Read the model definition and answer for the solid it produces. Units are mm, in the model's axes. Coordinates: 2 decimals unless noted, no trailing zeros. Loops run counter-clockwise (first coordinate to the right, second up) from the corner with the lowest first, then second, coordinate; pieces in that order, holes last.
from build123d import *

# Parameters (mm, degrees)
BOSS_EXTRUDE1_DEPTH          = 3
CUT_EXTRUDE_THIN1_DEPTH      = 73.819983521
CUT_EXTRUDE_THIN1_DEPTH_BACK = 3
FILLET1_R                    = 3.05
BOSS_EXTRUDE2_DEPTH          = 3
CUT_EXTRUDE1_DEPTH           = 77.32004979
CUT_EXTRUDE1_DEPTH_BACK      = 77.32004979
SKETCH4_R                    = 1.2
CUT_EXTRUDE_THIN2_DEPTH      = 77.32004979
CUT_EXTRUDE_THIN2_DEPTH_BACK = 3
FILLET2_R                    = 1.2
SKETCH6_W                    = 20
SKETCH6_H                    = 10
SKETCH6_R                    = 2.525
BOSS_EXTRUDE3_DEPTH          = 3
FILLET3_R                    = 3


with BuildPart() as part:
    # Sketch1 → Boss-Extrude1 (new body)
    with BuildSketch(Plane(origin=(0, 0, 0), x_dir=(1, 0, 0), z_dir=(0, 1, 0))):
        with BuildLine():
            Line((-27.5, 47.631397208), (-20.5, 35.507041555))
            ThreePointArc((-20.5, 35.507041555), (-40.649239316, 5.351573881), (-28.991378029, -28.991378029))
            Line((-28.991378029, -28.991378029), (-38.890872965, -38.890872965))
            ThreePointArc((-38.890872965, -38.890872965), (-54.529467376, 7.178940572), (-27.5, 47.631397208))
        make_face()
    extrude(amount=BOSS_EXTRUDE1_DEPTH)

    # Sketch2 → Cut-Extrude-Thin1 (cut, two sides: drawn at the far end of the back side and taken through both)
    with BuildSketch(Plane(origin=(0, 3, 0), x_dir=(1, 0, 0), z_dir=(0, 1, 0)).offset(-CUT_EXTRUDE_THIN1_DEPTH_BACK)):
        with BuildLine():
            ThreePointArc((-32.997630308, -29.03030992), (-43.925085447, -1.479651456), (-34.876429564, 26.743918204))
            Line((-34.876429564, 26.743918204), (-39.717071665, 30.455815838))
            ThreePointArc((-39.717071665, 30.455815838), (-50.021627455, -1.685018325), (-37.577506187, -33.0595452))
            Line((-37.577506187, -33.0595452), (-32.997630308, -29.03030992))
        make_face()
    extrude(amount=CUT_EXTRUDE_THIN1_DEPTH + CUT_EXTRUDE_THIN1_DEPTH_BACK, mode=Mode.SUBTRACT)

    # Fillet1
    fillet1_edges = [part.edges().sort_by_distance(p)[0] for p in [
        (-39.717071665, 1.5, -30.455815838),
        (-34.876429564, 1.5, -26.743918204),
        (-32.997630308, 1.5, 29.03030992),
        (-37.577506187, 1.5, 33.0595452),
    ]]
    fillet(fillet1_edges, radius=FILLET1_R - 0.0001)  # a hair under: the kernel refuses the full size

    # Sketch3 → Boss-Extrude2 (add)
    with BuildSketch(Plane(origin=(0, 0, 0), x_dir=(1, 0, 0), z_dir=(0, 1, 0))):
        with BuildLine():
            Line((-27.5, 47.631397208), (-30.5, 52.827549631))
            ThreePointArc((-30.5, 52.827549631), (-36.284189992, 49.035268498), (-41.601899964, 44.612575799))
            Line((-41.601899964, 44.612575799), (-37.509909803, 40.224453589))
            ThreePointArc((-37.509909803, 40.224453589), (-32.715253271, 44.212127334), (-27.5, 47.631397208))
        make_face()
    extrude(amount=BOSS_EXTRUDE2_DEPTH)

    # Sketch4 → Cut-Extrude1 (cut, two sides: drawn at the far end of the back side and taken through both)
    with BuildSketch(Plane(origin=(0, 3, 0), x_dir=(1, 0, 0), z_dir=(0, 1, 0)).offset(-CUT_EXTRUDE1_DEPTH_BACK)):
        with Locations(Location((-26.217006802, 39.609576548, 0), (0, 0, 270))):
            Circle(SKETCH4_R)
    extrude(amount=CUT_EXTRUDE1_DEPTH + CUT_EXTRUDE1_DEPTH_BACK, mode=Mode.SUBTRACT)

    # Sketch5 → Cut-Extrude-Thin2 (cut, two sides: drawn at the far end of the back side and taken through both)
    with BuildSketch(Plane(origin=(0, 3, 0), x_dir=(1, 0, 0), z_dir=(0, 1, 0)).offset(-CUT_EXTRUDE_THIN2_DEPTH_BACK)):
        with BuildLine():
            ThreePointArc((-30.458263972, 49.433106342), (-34.605510743, 46.252091255), (-36.751172642, 41.486102609))
            Line((-36.751172642, 41.486102609), (-34.388369089, 41.065199567))
            ThreePointArc((-34.388369089, 41.065199567), (-32.723977149, 44.762181415), (-29.506953953, 47.22969779))
            Line((-29.506953953, 47.22969779), (-30.458263972, 49.433106342))
        make_face()
    extrude(amount=CUT_EXTRUDE_THIN2_DEPTH + CUT_EXTRUDE_THIN2_DEPTH_BACK, mode=Mode.SUBTRACT)

    # Fillet2
    fillet2_edges = [part.edges().sort_by_distance(p)[0] for p in [
        (-34.388369089, 1.5, -41.065199567),
        (-36.751172642, 1.5, -41.486102609),
        (-30.458263972, 1.5, -49.433106342),
        (-29.506953953, 1.5, -47.22969779),
    ]]
    fillet(fillet2_edges, radius=FILLET2_R - 0.0001)  # a hair under: the kernel refuses the full size

    # Sketch6 → Boss-Extrude3 (add)
    with BuildSketch(Plane(origin=(0, 0, 0), x_dir=(1, 0, 0), z_dir=(0, 1, 0))):
        with Locations((-64.772255751, 0)):
            Rectangle(SKETCH6_W, SKETCH6_H)
        with Locations(Location((-70.772255751, 0, 0), (0, 0, 90))):
            Circle(SKETCH6_R, mode=Mode.SUBTRACT)
        with Locations(Location((-60.772255751, 0, 0), (0, 0, 90))):
            Circle(SKETCH6_R, mode=Mode.SUBTRACT)
    extrude(amount=BOSS_EXTRUDE3_DEPTH)

    # Fillet3
    fillet3_edges = [part.edges().sort_by_distance(p)[0] for p in [
        (-74.772255751, 1.5, 5),
        (-74.772255751, 1.5, -5),
        (-54.772255751, 1.5, 5),
        (-54.772255751, 1.5, -5),
        (-37.509909803, 1.5, -40.224453589),
        (-41.601899964, 1.5, -44.612575799),
        (-30.5, 1.5, -52.827549631),
        (-20.5, 1.5, -35.507041555),
        (-28.991378029, 1.5, 28.991378029),
        (-38.890872965, 1.5, 38.890872965),
    ]]
    fillet(fillet3_edges, radius=FILLET3_R - 0.0001)  # a hair under: the kernel refuses the full size


solid = part.part
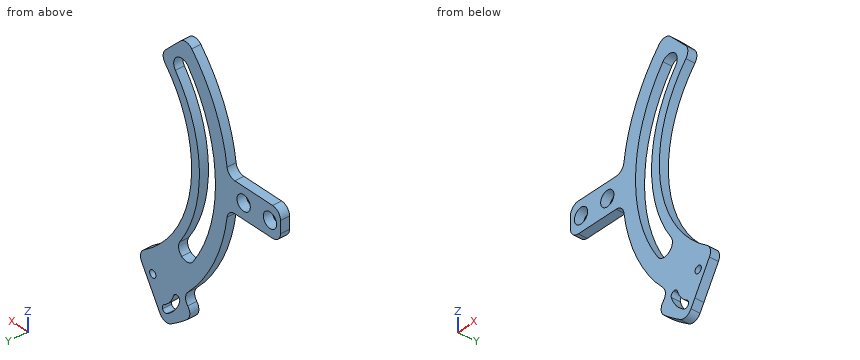
Item 1: Given pin 1 (1.5 mm diameter, centred on y = 1, z = 12.5, fed in from -X); pin 2 (10 mm diameter, centred on x = -66.5, z = -8.5, fed in from -Y); pin 3 (0.9 mm diameter, centred on x = -65.5, y = 1, fed in from +Z), each flat-ended and moving along its own axis, determine where each tip first touches the part or whether it passes through.
Numbers:
pin 1: stops at x = -53.73
pin 2: stops at y = 0
pin 3: stops at z = 5
Item 2: Find the intervals of material crossed by line 1 along X through (y, z) = (0.65, 0); line 2 along Z through (x, y) = (-31.5, 2.35); line 3 along Z through (x, y) = (-30.5, 0.35), in increasing order.
Numbers:
line 1: x = -74.77 to -73.3, -68.25 to -63.3, -58.25 to -50.05, -43.95 to -41
line 2: z = -51.66 to -48.9, -46.01 to -26.24, 26.24 to 31.5
line 3: z = -51.47 to -48.85, -46.72 to -27.4, 27.53 to 30.3
Item 3: A cutting plane is placed at A-A on z = 0. Determine the outline of the cut face in (x, y).
Numbers:
outline: (-74.77, 0) - (-73.3, 0) - (-73.3, 3) - (-74.77, 3) - close; (-68.25, 0) - (-63.3, 0) - (-63.3, 3) - (-68.25, 3) - close; (-58.25, 0) - (-50.05, 0) - (-50.05, 3) - (-58.25, 3) - close; (-43.95, 0) - (-41, 0) - (-41, 3) - (-43.95, 3) - close
Item 4: A cutting plane is placed at C-C on y = 0.85. Give the number of separate pieces and of enclosed holes in the cut face, then the cut area to 3 significant figures.
Numbers:
separate pieces: 1
enclosed holes: 5
area: 1,050 mm2
Item 5: A cutting plane is placed at B-B on z = -20.5. Determine the outline of the cut face in (x, y), then the cut area to 3 significant figures.
Numbers:
outline: (-51.04, 0) - (-45.66, 0) - (-45.66, 3) - (-51.04, 3) - close; (-38.88, 0) - (-35.51, 0) - (-35.51, 3) - (-38.88, 3) - close
area: 26.2 mm2
